Geometry: final body of the model. Coordinates: model frame, mm. A direction names the side the tool comes from. Round coordinates to 2 decimals unless told otherwise and drop trailing zeros. Write each loop counter-clockwise with the first axis right and the second up, starting at its lowest first coordinate (ties: lowest second). Pieces come first, ordered by that corner, then holes. Notation, with made-up numbers: (83, 26.25) -> (87, 26.25) arc R18 ccw to (87, 41.25) -> close; hole circle Ø4 at (27, 8). An arc over 180 degrees is marked (long way). Use one line per item in the form item = value. Start each with the question number.
1. Line query: L1, parallel to X at y = 9, z = 24; L2, parallel to Z at x = 23.4, y = 8.25; L3, parallel to Y at x = 4, z = 11.5. Output: solid intervals per line, ascending.
2. Reachability of faces 5 (the face through (28, 15.5, 19.5)), 6 (the face through (1.345, 1.373, 38.007)), 7 (the face through (14, 2, 25)), 8 (the face through (24.55, 8, 7)), 9 (the face through (9.59, 0.99, 10.78)) from +Z, -Z, +X, -X, +Y, -Y: full face, straight path, thin tool, end or side. Return the list, or none.
3. Cut plane C-C, the plane x = 9.25. Return the cut outline in (y, z).
4. Cut plane A-A, the plane y = 8.25. Return the cut outline in (x, z) (3 decimals), plus the area to 3 significant figures.
5. Draft query along Y for faces 1 (the face through (26.744, 8.211, 5.754)), 2 (the face through (1, 1, 20)), 3 (the face through (1.55, 14.93, 1.21)), 4 (the face through (2, 8, 21)). Return one class per face: pulls with the +Y half, pulls with the -Y half, needs draft (parallel to the pull), parting line crosses it, or undercut.
6. Cut plane B-B, the plane z = 27.5. Return the cut outline in (x, y).
7. Pin query (flat end, axial travel): pin 1 Ø2 at (y, z) = (16, 7) entering from +X; pin 2 Ø6 at (x, y) = (9, 6.5) entering from +Z; pin 3 Ø5 at (x, y) = (26, 9.5) entering from +Z; pin 4 Ø1.3 at (y, z) = (8.25, 9) entering from +X. Return the tip coordinate at first contact, or that it passes through.
```python
from build123d import *

# Parameters (mm, degrees)
F0_W      = 29
F0_H      = 16.5
F1_DEPTH  = 38.5
F2_T      = -2
F3_DEPTH  = 2.25
F4_SIZE   = 2
F5_SIZE   = 2
F6_SIZE   = 1
F8_DEPTH  = 16.501
F9_W      = 7.54
F9_H      = 7.25
F9_R      = 1.1
F10_DEPTH = 6.35
F11_W     = 5.538
F11_H     = 5.53
F13_W     = 5.538
F13_H     = 4.583


with BuildPart() as f1:
    # F0 (on Top) → F1 (new body)
    with BuildSketch(Plane.XY):
        with Locations((14.5, 8.25)):
            Rectangle(F0_W, F0_H)
    extrude(amount=F1_DEPTH)

    # F2
    f2_openings = [f1.faces().sort_by_distance(p)[0] for p in [
        (14.5, 8.25, 38.5),
    ]]
    offset(amount=F2_T, openings=f2_openings)

    # F3 (add): a face of the model
    f3_faces = [f1.faces().sort_by_distance(p)[0] for p in [
        (14.5, 8.25, 2),
    ]]
    extrude(f3_faces, amount=F3_DEPTH)

    # F4
    f4_edges = [f1.edges().sort_by_distance(p)[0] for p in [
        (29, 16.5, 19.25),
        (29, 0, 19.25),
        (0, 16.5, 19.25),
        (0, 0, 19.25),
    ]]
    chamfer(f4_edges, length=F4_SIZE)

    # F5
    f5_edges = [f1.edges().sort_by_distance(p)[0] for p in [
        (0, 8.25, 0),
        (1, 15.5, 0),
        (1, 1, 0),
        (14.5, 16.5, 0),
        (14.5, 0, 0),
        (28, 15.5, 0),
        (28, 1, 0),
        (29, 8.25, 0),
    ]]
    chamfer(f5_edges, length=F5_SIZE)

    # F6
    f6_edges = [f1.edges().sort_by_distance(p)[0] for p in [
        (14.5, 0, 38.5),
        (1, 1, 38.5),
        (0, 8.25, 38.5),
        (1, 15.5, 38.5),
        (14.5, 16.5, 38.5),
        (28, 15.5, 38.5),
        (29, 8.25, 38.5),
        (28, 1, 38.5),
    ]]
    chamfer(f6_edges, length=F6_SIZE)

    # F7 (on face) → F8 (cut, through all)
    with BuildSketch(Plane.XZ):
        Polygon((17.365, 12.834), (12.635, 12.834), (6.464, 8.667), (6.464, 4.94), (23.536, 4.94), (23.536, 8.667), align=None)
    extrude(amount=-F8_DEPTH, mode=Mode.SUBTRACT)

    # F9 (on face) → F10 (join)
    with BuildSketch(Plane.YZ.offset(29)):
        with Locations((8.25, 7.875)):
            Rectangle(F9_W, F9_H)
        with Locations((8.25, 9)):
            Circle(F9_R, mode=Mode.SUBTRACT)
    extrude(amount=-F10_DEPTH)

    # F11 (on face) → F14 section 0
    with BuildSketch(Plane.YZ.offset(29)):
        with Locations((8.25, 8.037)):
            Rectangle(F11_W, F11_H)
    # F13 (on offset) → F14 section 1
    with BuildSketch(Plane.YZ.offset(24.55)):
        with Locations((8.25, 8.5135)):
            Rectangle(F13_W, F13_H)
    loft(mode=Mode.SUBTRACT)


solid = f1.part
```
Outcome:
q1.L1 = 0 to 2, 27 to 29
q1.L2 = 0 to 7.9, 10.1 to 11.5
q1.L3 = 0 to 2, 14.5 to 16.5
q2.face_5 = +Z, -Z, +X, +Y
q2.face_6 = +Z, -X, -Y
q2.face_7 = +Z
q2.face_8 = +X
q2.face_9 = +Y, -Y
q3.outline = (0, 2) -> (2, 0) -> (14.5, 0) -> (16.5, 2) -> (16.5, 4.94) -> (14.5, 4.94) -> (14.5, 4.25) -> (2, 4.25) -> (2, 4.94) -> (0, 4.94) -> close; (0, 10.55) -> (2, 10.55) -> (2, 38.5) -> (1, 38.5) -> (0, 37.5) -> close; (14.5, 10.55) -> (16.5, 10.55) -> (16.5, 37.5) -> (15.5, 38.5) -> (14.5, 38.5) -> close
q4.outline = (0, 2) -> (2, 0) -> (27, 0) -> (29, 2) -> (29, 5.272) -> (24.55, 6.222) -> (24.55, 7.9) -> (22.65, 7.9) -> (22.65, 4.25) -> (2, 4.25) -> (2, 38.5) -> (1, 38.5) -> (0, 37.5) -> close; (22.65, 10.1) -> (24.55, 10.1) -> (24.55, 10.805) -> (29, 10.802) -> (29, 37.5) -> (28, 38.5) -> (27, 38.5) -> (27, 11.5) -> (22.65, 11.5) -> close
q4.area = 260 mm^2
q5.face_1 = undercut
q5.face_2 = pulls with the -Y half
q5.face_3 = pulls with the +Y half
q5.face_4 = undercut
q6.outline = (0, 2) -> (2, 0) -> (27, 0) -> (29, 2) -> (29, 14.5) -> (27, 16.5) -> (2, 16.5) -> (0, 14.5) -> close; hole (2, 2) -> (27, 2) -> (27, 14.5) -> (2, 14.5) -> close
q7.pin_1 = 28.5
q7.pin_2 = 4.25
q7.pin_3 = 38.5
q7.pin_4 = 2
